from build123d import *

# Parameters (mm, degrees)
CROQUIS_BASE_W           = 54
CROQUIS_BASE_H           = 20
SALIENTE_EXTRUIR1_DEPTH  = 2.6
CORTAR_EXTRUIR1_DEPTH    = 2.6
CROQUIS_STEP_2_3_W       = 40
CROQUIS_STEP_2_3_H       = 20
SALIENTE_EXTRUIR2_DEPTH  = 6.9
SALIENTE_EXTRUIR5_DEPTH  = 2
CROQUIS5_W               = 7
CROQUIS5_H               = 1.2
SALIENTE_EXTRUIR6_DEPTH  = 2
CROQUIS3_W               = 7
CROQUIS3_H               = 1.2
SALIENTE_EXTRUIR7_DEPTH  = 2
CORTAR_EXTRUIR4_DEPTH    = 1.2
CORTAR_EXTRUIR5_DEPTH    = 1.2
CROQUIS10_R              = 6.75
SALIENTE_EXTRUIR8_DEPTH  = 0.8
CROQUIS11_R              = 5.5
SALIENTE_EXTRUIR9_DEPTH  = 0.55
CHAFL_N1_START           = 18.526197667
CHAFL_N1_OUTLINE_W       = 2.828427125
CHAFL_N1_OUTLINE_H       = 18.6
CHAFL_N1_DEPTH           = 2.473802333
CROQUIS12_R              = 2.95
SALIENTE_EXTRUIR10_DEPTH = 4


with BuildPart() as part:
    # Croquis base → Saliente-Extruir1 (new body)
    with BuildSketch(Plane(origin=(0, 0, 0), x_dir=(1, 0, 0), z_dir=(0, 1, 0))):
        Rectangle(CROQUIS_BASE_W, CROQUIS_BASE_H)
    extrude(amount=SALIENTE_EXTRUIR1_DEPTH)

    # Croquis step 2 → Cortar-Extruir1 (cut)
    with BuildSketch(Plane(origin=(0, 2.6, 0), x_dir=(1, 0, 0), z_dir=(0, 1, 0))):
        with BuildLine():
            Line((-26.204050808, 5.88), (-27, 5.88))
            Line((-27, 5.88), (-27, 3.88))
            Line((-27, 3.88), (-26.204050808, 3.88))
            ThreePointArc((-26.204050808, 3.88), (-22.472, 4.88), (-26.204050808, 5.88))
        make_face()
        with BuildLine():
            Line((-26.204050808, -3.88), (-27, -3.88))
            Line((-27, -3.88), (-27, -5.88))
            Line((-27, -5.88), (-26.204050808, -5.88))
            ThreePointArc((-26.204050808, -5.88), (-22.472, -4.88), (-26.204050808, -3.88))
        make_face()
        with BuildLine():
            Line((26.204050808, 3.88), (27, 3.88))
            Line((27, 3.88), (27, 5.88))
            Line((27, 5.88), (26.204050808, 5.88))
            ThreePointArc((26.204050808, 5.88), (22.472, 4.88), (26.204050808, 3.88))
        make_face()
        with BuildLine():
            Line((26.204050808, -5.88), (27, -5.88))
            Line((27, -5.88), (27, -3.88))
            Line((27, -3.88), (26.204050808, -3.88))
            ThreePointArc((26.204050808, -3.88), (22.472, -4.88), (26.204050808, -5.88))
        make_face()
    extrude(amount=-CORTAR_EXTRUIR1_DEPTH, mode=Mode.SUBTRACT)

    # Croquis step 2<3> → Saliente-Extruir2 (add)
    with BuildSketch(Plane(origin=(0, 2.6, 0), x_dir=(1, 0, 0), z_dir=(0, 1, 0))):
        Rectangle(CROQUIS_STEP_2_3_W, CROQUIS_STEP_2_3_H)
    extrude(amount=SALIENTE_EXTRUIR2_DEPTH)

    # Croquis7 → Saliente-Extruir5 (add)
    with BuildSketch(Plane(origin=(0, 9.5, 0), x_dir=(1, 0, 0), z_dir=(0, 1, 0))):
        with BuildLine():
            Line((-10, 9.3), (16.7, 9.3))
            Line((16.7, 9.3), (16.7, -9.3))
            Line((16.7, -9.3), (-10, -9.3))
            ThreePointArc((-10, -9.3), (-19.3, 0), (-10, 9.3))
        make_face()
    extrude(amount=SALIENTE_EXTRUIR5_DEPTH)

    # Croquis5 → Saliente-Extruir6 (add)
    with BuildSketch(Plane(origin=(0, 2.6, 0), x_dir=(1, 0, 0), z_dir=(0, 1, 0))):
        with Locations((23.5, 0)):
            Rectangle(CROQUIS5_W, CROQUIS5_H)
    extrude(amount=SALIENTE_EXTRUIR6_DEPTH)

    # Croquis3 → Saliente-Extruir7 (add)
    with BuildSketch(Plane(origin=(0, 2.6, 0), x_dir=(1, 0, 0), z_dir=(0, 1, 0))):
        with Locations((-23.5, 0)):
            Rectangle(CROQUIS3_W, CROQUIS3_H)
    extrude(amount=SALIENTE_EXTRUIR7_DEPTH)

    # Croquis8 → Cortar-Extruir4 (cut)
    with BuildSketch(Plane.XY.offset(0.6)):
        Polygon((-27, 2.6), (-27, 4.6), (-20, 4.6), align=None)
    extrude(amount=-CORTAR_EXTRUIR4_DEPTH, mode=Mode.SUBTRACT)

    # Croquis9 → Cortar-Extruir5 (cut)
    with BuildSketch(Plane.XY.offset(0.6)):
        Polygon((27, 2.6), (20, 4.6), (27, 4.6), align=None)
    extrude(amount=-CORTAR_EXTRUIR5_DEPTH, mode=Mode.SUBTRACT)

    # Croquis10 → Saliente-Extruir8 (add)
    with BuildSketch(Plane(origin=(0, 11.5, 0), x_dir=(1, 0, 0), z_dir=(0, 1, 0))):
        with Locations(Location((-10, 0, 0), (0, 0, 270))):
            Circle(CROQUIS10_R)
    extrude(amount=SALIENTE_EXTRUIR8_DEPTH)

    # Croquis11 → Saliente-Extruir9 (add)
    with BuildSketch(Plane(origin=(0, 12.3, 0), x_dir=(1, 0, 0), z_dir=(0, 1, 0))):
        with Locations(Location((-10, 0, 0), (0, 0, 270))):
            Circle(CROQUIS11_R)
    extrude(amount=SALIENTE_EXTRUIR9_DEPTH)

    # Chaflán1: read off the stored shape, not the designer's step
    # Chaflán1 outline → Chaflán1 (cut)
    with BuildSketch(Plane(origin=(0, 0, 0), x_dir=(0.707106781186548, -0.707106781186547, 0), z_dir=(0.707106781186547, 0.707106781186548, 0)).offset(CHAFL_N1_START)):
        with Locations((3.676955263, 0)):
            Rectangle(CHAFL_N1_OUTLINE_W, CHAFL_N1_OUTLINE_H)
    extrude(amount=CHAFL_N1_DEPTH, mode=Mode.SUBTRACT)

    # Croquis12 → Saliente-Extruir10 (add)
    with BuildSketch(Plane(origin=(0, 12.85, 0), x_dir=(1, 0, 0), z_dir=(0, 1, 0))):
        with Locations(Location((-10, 0, 0), (0, 0, 270))):
            Circle(CROQUIS12_R)
    extrude(amount=SALIENTE_EXTRUIR10_DEPTH)


solid = part.part
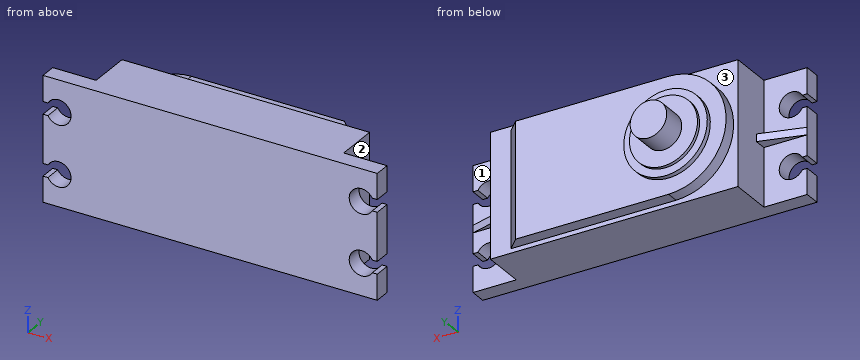
The listing builds one solid part. Answer for the finished solid, in the listing's coordinates (mm). Face numbers are marked on the shaded views. A direction names the side the tool comes from. Give positions to 0.01 mm unless a question says otherwise; leave off trailing zeros. Loops run counter-clockwise (first coordinate to the right, second up) from the corner with the lowest first, then second, coordinate; pieces in that order, holes last. Notation, with made-up numbers: M 88,28.5 L 115,28.5 A21 ccw 115,52.5 Z; hole C 89,71.5 d10. An arc over 180 degrees is marked long. Answer as CSV lines item,"result".
Item 1: Given pin 1 Ø0.6 at (x, y) = (6, 11) entering from -Z; pin 2 Ø10 at (x, z) = (-5, -2.5) entering from +Y; pin 3 Ø7.5 at (x, z) = (23, -6) entering from +Y; pin 4 Ø3.5 at (x, z) = (-23.5, -6.5) entering from +Y, each flat-ended and moving along its own axis, determine where each tip first touches the part or whether it passes through.
Values follow:
pin 1,"stops at z = -9.3"
pin 2,"stops at y = 16.85"
pin 3,"stops at y = 9.5"
pin 4,"stops at y = 2.6"
Item 2: The part is cut by section D-D (z = -2.25). Give the vertices of the cut face in (x, y).
Values follow:
outline,"M -27,0 L 27,0 L 27,2.6 L 20,2.6 L 20,9.5 L 16.7,9.5 L 14.7,11.5 L -3.64,11.5 L -3.64,12.3 L -4.98,12.3 L -4.98,12.85 L -8.09,12.85 L -8.09,16.85 L -11.91,16.85 L -11.91,12.85 L -15.02,12.85 L -15.02,12.3 L -16.36,12.3 L -16.36,11.5 L -19.02,11.5 L -19.02,9.5 L -20,9.5 L -20,2.6 L -27,2.6 Z"
Item 3: Which of the six approach directions +Z, -Z, +X, -X, +Y, -Y give full straight-line access (tool end or side, diameter ignored) to the marked faces 1, 2 and 3?
Values follow:
face 1,"+Z, +X, +Y"
face 2,"+X, +Y"
face 3,"+Y"
Item 4: The part is cut by section B-B (y = 1.75). Give the vertices of the cut face in (x, z), and give its area (3 significant figures).
Values follow:
outline,"M -27,-10 L 27,-10 L 27,-5.88 L 26.2,-5.88 A2 cw long 26.2,-3.88 L 27,-3.88 L 27,3.88 L 26.2,3.88 A2 cw long 26.2,5.88 L 27,5.88 L 27,10 L -27,10 L -27,5.88 L -26.2,5.88 A2 cw long -26.2,3.88 L -27,3.88 L -27,-3.88 L -26.2,-3.88 A2 cw long -26.2,-5.88 L -27,-5.88 Z"
area,"1,020 mm^2"
Item 5: The part is cut by section A-A (z = 0). Give the vertices of the cut face in (x, y).
Values follow:
outline,"M -27,0 L 27,0 L 27,2.6 L 20,4.6 L 20,9.5 L 16.7,9.5 L 14.7,11.5 L -3.25,11.5 L -3.25,12.3 L -4.5,12.3 L -4.5,12.85 L -7.05,12.85 L -7.05,16.85 L -12.95,16.85 L -12.95,12.85 L -15.5,12.85 L -15.5,12.3 L -16.75,12.3 L -16.75,11.5 L -19.3,11.5 L -19.3,9.5 L -20,9.5 L -20,4.6 L -27,2.6 Z"
Item 6: The part is cut by section C-C (x = 12.5). Give the vertices of the cut face in (y, z), and give its area (3 significant figures).
Values follow:
outline,"M 0,-10 L 9.5,-10 L 9.5,-9.3 L 11.5,-9.3 L 11.5,9.3 L 9.5,9.3 L 9.5,10 L 0,10 Z"
area,"227 mm^2"
Item 7: Straight lines are drawn through the part: line 1 along X through (y, z) = (4.5, -4.75); line 2 along Y through (x, z) = (22, 7.25); line 3 along X through (y, z) = (0.9, 4.88). For each, find the intervals that lie inside material, in ascending order. Write a range as [from, to].
Values follow:
line 1,"x = [-20, 20]"
line 2,"y = [0, 2.6]"
line 3,"x = [-22.47, 22.47]"
